Work out the finished part from the listing and answer in its coordinate system (mm). Round coordinates to 2 decimals unless told otherwise and drop trailing zeros. Order: outer loops, then holes, each group sorted by start corner. A loop starts at its lowest first (then second) coordinate and runs counter-clockwise, first axis right, second up. Notation, with made-up numbers: (-3.75, -34) - (6.25, -34) arc R32 cw to (6.25, -2) - close; hole circle Ø9 at (-3, 53). An arc over 180 degrees is marked (long way). Answer in a Markdown table with one row per item.
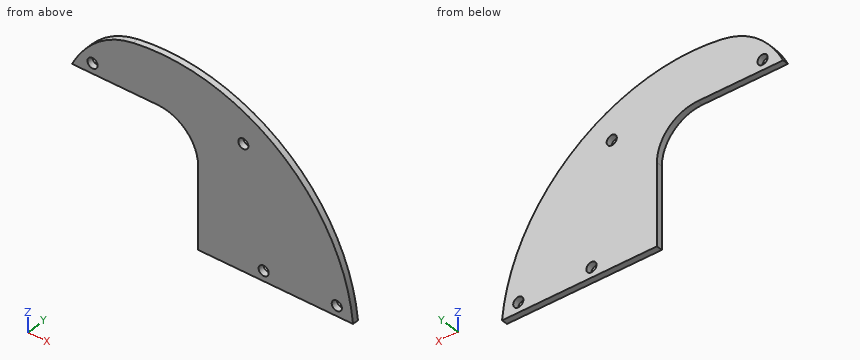
from build123d import *

# Parameters (mm, degrees)
PCB_BOARD_DEPTH     = 0.75
BOSS_EXTRUDE1_DEPTH = 1.5
SKETCH5_R           = 1.25
MOUTING_HOLES_DEPTH = 10


with BuildPart() as part:
    # Sketch1 → Pcb Board (new, symmetric)
    with BuildSketch(Plane(origin=(0, 0, 0), x_dir=(1, 0, 0), z_dir=(0, 1, 0))):
        with BuildLine():
            ThreePointArc((-33.016678433, -25.226747869), (3.126055598, -15.93137563), (21.101274409, 16.773252131))
            Line((21.101274409, 16.773252131), (-17.016678433, 16.773252131))
            Line((-17.016678433, 16.773252131), (-17.016678433, -3.226747869))
            ThreePointArc((-17.016678433, -3.226747869), (-19.945610621, -10.297815681), (-27.016678433, -13.226747869))
            Line((-27.016678433, -13.226747869), (-43.016678433, -13.226747869))
            Line((-43.016678433, -13.226747869), (-43.016678432, -20.226747869))
            ThreePointArc((-43.016678433, -20.226747869), (-38.403625629, -23.500642262), (-33.016678433, -25.226747869))
        make_face()
    extrude(amount=PCB_BOARD_DEPTH, both=True)

    # Sketch6 → Boss-Extrude1 (add)
    with BuildSketch(Plane(origin=(0, 0.75, 0), x_dir=(1, 0, 0), z_dir=(0, 1, 0))):
        with BuildLine():
            Line((-43.016678433, -13.226747869), (-48.055127106, -13.226747869))
            ThreePointArc((-48.055127106, -13.226747869), (-45.844966452, -16.949205227), (-43.016678433, -20.226747869))
            Line((-43.016678433, -20.226747869), (-43.016678433, -13.226747869))
        make_face()
    extrude(amount=-BOSS_EXTRUDE1_DEPTH)

    # Sketch5 → Mouting Holes (cut)
    with BuildSketch(Plane(origin=(0, 0.75, 0), x_dir=(1, 0, 0), z_dir=(0, 1, 0))):
        with Locations(Location((-43.016678433, -15.726747869, 0), (0, 0, 270))):
            Circle(SKETCH5_R)
        with Locations(Location((17.101274409, 14.273252131, 0), (0, 0, 270))):
            Circle(SKETCH5_R)
        with Locations(Location((-5.898725591, -13.726747869, 0), (0, 0, 270))):
            Circle(SKETCH5_R)
        with Locations(Location((-0.898725591, 14.273252131, 0), (0, 0, 270))):
            Circle(SKETCH5_R)
    extrude(amount=-MOUTING_HOLES_DEPTH, mode=Mode.SUBTRACT)


solid = part.part
1) Each of these flat-tipped pins is pushed along its axis until it touches: pin 1 (4 mm diameter, centred on x = -43.02, z = 15.73, fed in from -Y); pin 2 (0.8 mm diameter, centred on x = -41, y = -0.5, fed in from -Z). Where does it stop, or does it pass through?
Filled in:
| item | result |
|---|---|
| pin 1 | stops at y = -0.75 |
| pin 2 | stops at z = 13.23 |
2) Find section B-B, the plane z = 10. Give the vertices of the cut face in (x, y), then the cut area to 3 significant figures.
Filled in:
| item | result |
|---|---|
| outline | (-19.66, -0.75) - (9.46, -0.75) - (9.46, 0.75) - (-19.66, 0.75) - close |
| area | 43.7 mm^2 |
3) Find the intervals of material crossed by probe 1 along Z at (x, y) = (16, 0.6); probe 2 along Z at (x, y) = (-33, -0.3); probe 3 along X at (y, z) = (-0.6, 20), in increasing order. Write a range as from..to.
Filled in:
| item | result |
|---|---|
| probe 1 | z = -16.77..-14.86, -13.68..0.5 |
| probe 2 | z = 13.23..25.23 |
| probe 3 | x = -43.25..-3.07 |
4) Find section C-C, the plane x = -13. Give the vertices of the cut face in (y, z).
Filled in:
| item | result |
|---|---|
| outline | (-0.75, -16.77) - (0.75, -16.77) - (0.75, 24.06) - (-0.75, 24.06) - close |
5) Find section A-A, the plane y = -0.45. Give the vertices of the cut face in (x, z), then the cut area to 3 significant figures.
Filled in:
| item | result |
|---|---|
| outline | (-48.06, 13.23) - (-27.02, 13.23) arc R10 cw to (-17.02, 3.23) - (-17.02, -16.77) - (21.1, -16.77) arc R47 ccw to (-33.02, 25.23) arc R18.49 ccw to (-43.02, 20.23) arc R24.61 ccw to start; hole circle Ø2.5 at (-43.02, 15.73); hole circle Ø2.5 at (-5.9, 13.73); hole circle Ø2.5 at (-0.9, -14.27); hole circle Ø2.5 at (17.1, -14.27) |
| area | 1,480 mm^2 |
